Can you work these out from the model? Positions are in its coordinate system, mm. A direction names the side the tool comes from. Round coordinates to 2 decimals unless told otherwise and drop trailing zeros. Order: outer loops, then holes, each group sorted by start corner. A loop starts at its lowest first (then second) coordinate and runs counter-clockwise, first axis right, second up. Notation, with made-up numbers: (-5.5, 75) -> (32.5, 75) arc R22 cw to (32.5, 88) -> close; hole circle Ø2 at (-26, -11.5). An arc over 180 degrees is marked (long way). One line per item, written item: value.
```python
from build123d import *

# Parameters (mm, degrees)
SKETCH1_R           = 2
EXTRUDE1_DEPTH      = 8
CUT_SWEEP1_PITCH    = 0.7
SKETCH6_R           = 3.5
EXTRUDE2_DEPTH      = 4
CUT_EXTRUDE1_DEPTH  = 2.25
CHAMFER1_SIZE       = 0.35
SKETCH10_R          = 2
BOSS_EXTRUDE1_DEPTH = 8
CHAMFER2_SIZE       = 0.5
CHAMFER2_SIZE2      = 0.866025404


with BuildPart() as part:
    # Sketch1 → Extrude1 (new body)
    with BuildSketch(Plane.XY):
        Circle(SKETCH1_R)
    extrude(amount=-EXTRUDE1_DEPTH)

    # Cut-Sweep1: the profile of Sketch3 profile screwed along a right-hand helix of 12.428571 turns, 6 arcs to a turn; built about Z, then put on its axis
    cut_sweep1_z = Axis((0, 0, 0), (0, 0, 1))
    cut_sweep1_corners = [(2.0003, 0, -0.612673205), (1.545336663, 0, -0.35), (1.545336663, 0, -0.2625), (2.0003, 0, 0.000173205)]
    with BuildLine(mode=Mode.PRIVATE) as cut_sweep1_profile:
        Line(cut_sweep1_corners[0], cut_sweep1_corners[1])
        Line(cut_sweep1_corners[1], cut_sweep1_corners[2])
        Line(cut_sweep1_corners[2], cut_sweep1_corners[3])
        Line(cut_sweep1_corners[3], cut_sweep1_corners[0])
    cut_sweep1_cap = Face(cut_sweep1_profile.wire())
    cut_sweep1_turn_angles = [0, 30, 60, 90, 120, 150, 180, 210, 240, 270, 300, 330, 360]
    cut_sweep1_turn_weights = [1, 0.8660254037844387, 1, 0.8660254037844387, 1, 0.8660254037844387, 1, 0.8660254037844387, 1, 0.8660254037844387, 1, 0.8660254037844387, 1]
    cut_sweep1_turn_rails = [Edge.make_bspline([Vector(p[0], p[1], 0).rotate(cut_sweep1_z, cut_sweep1_turn_angles[k]) / cut_sweep1_turn_weights[k] + Vector(0, 0, p[2] + CUT_SWEEP1_PITCH * cut_sweep1_turn_angles[k] / 360) for k in range(13)], [0, 0, 0, 1, 1, 2, 2, 3, 3, 4, 4, 5, 5, 6, 6, 6], 2, cut_sweep1_turn_weights) for p in cut_sweep1_corners]
    cut_sweep1_turn_sides = [Face.make_surface_from_curves(cut_sweep1_turn_rails[p[0]], cut_sweep1_turn_rails[p[1]]) for p in [(0, 1), (1, 2), (2, 3), (3, 0)]]
    cut_sweep1_last_angles = [4320, 4350, 4380, 4410, 4440, 4457.142857143, 4474.285714286]
    cut_sweep1_last_weights = [1, 0.8660254037844387, 1, 0.8660254037844387, 1, 0.9555728057861561, 1]
    cut_sweep1_last_rails = [Edge.make_bspline([Vector(p[0], p[1], 0).rotate(cut_sweep1_z, cut_sweep1_last_angles[k]) / cut_sweep1_last_weights[k] + Vector(0, 0, p[2] + CUT_SWEEP1_PITCH * cut_sweep1_last_angles[k] / 360) for k in range(7)], [0, 0, 0, 1, 1, 2, 2, 3, 3, 3], 2, cut_sweep1_last_weights) for p in cut_sweep1_corners]
    cut_sweep1_last_sides = [Face.make_surface_from_curves(cut_sweep1_last_rails[p[0]], cut_sweep1_last_rails[p[1]]) for p in [(0, 1), (1, 2), (2, 3), (3, 0)]]
    cut_sweep1 = Plane(origin=(0, 0, 0), x_dir=(0, 1, 0), z_dir=(0, 0, -1)) * Solid(Shell([*[p.moved(Location((0, 0, CUT_SWEEP1_PITCH * i))) for i in range(12) for p in cut_sweep1_turn_sides], *cut_sweep1_last_sides, cut_sweep1_cap, cut_sweep1_cap.rotate(cut_sweep1_z, 4474.285714286).moved(Location((0, 0, CUT_SWEEP1_PITCH * 4474.285714286 / 360)))]))
    add(cut_sweep1, mode=Mode.SUBTRACT)

    # Sketch4 → Cut-Revolve1 (revolve, cut)
    with BuildSketch(Plane(origin=(0, 0, 0), x_dir=(0, 0, -1), z_dir=(1, 0, 0)), mode=Mode.PRIVATE) as cut_revolve1_sk:
        Polygon((0.496211411, 2), (0, 1.291336663), (0, 2), align=None)
    revolve(cut_revolve1_sk.sketch.rotate(Axis((0, 0, 0), (0, 0, -1)), 271.401126896), axis=Axis((0, 0, 0), (0, 0, -1)), mode=Mode.SUBTRACT)

    # Sketch6 → Extrude2 (add)
    with BuildSketch(Plane(origin=(0, 0, -8), x_dir=(-1, 0, 0), z_dir=(0, 0, -1))):
        Circle(SKETCH6_R)
    extrude(amount=EXTRUDE2_DEPTH)

    # Sketch7 → Cut-Extrude1 (cut)
    with BuildSketch(Plane(origin=(0, 0, -12), x_dir=(-1, 0, 0), z_dir=(0, 0, -1))):
        Polygon((0, 1.732050808), (-1.5, 0.866025404), (-1.5, -0.866025404), (0, -1.732050808), (1.5, -0.866025404), (1.5, 0.866025404), align=None)
    extrude(amount=-CUT_EXTRUDE1_DEPTH, mode=Mode.SUBTRACT)

    # Cut-Extrude2 cone 1 section (through the dimple's axis) → Cut-Extrude2 (revolve, cut)
    with BuildSketch(Plane(origin=(0, 0, -12), x_dir=(0, 1, 0), z_dir=(1, 0, 0))):
        Polygon((0, 0), (1.732050808, 0), (0, 1.732050808), align=None)
    revolve(axis=Axis((0, 0, -12), (0, 0, 1)), mode=Mode.SUBTRACT)

    # Chamfer1
    chamfer1_edges = [part.edges().sort_by_distance(p)[0] for p in [
        (3.5, 0, -8),
        (3.5, 0, -12),
    ]]
    chamfer(chamfer1_edges, length=CHAMFER1_SIZE)

    # Sketch10 → Boss-Extrude1 (add)
    with BuildSketch(Plane.XY):
        Circle(SKETCH10_R)
    extrude(amount=-BOSS_EXTRUDE1_DEPTH)

    # Chamfer2
    chamfer2_edges = [part.edges().sort_by_distance(p)[0] for p in [
        (-2, 0, 0),
    ]]
    chamfer2_side = [part.faces().sort_by_distance(p)[0] for p in [
        (-2, 0, -4),
    ]]
    chamfer(chamfer2_edges, length=CHAMFER2_SIZE, length2=CHAMFER2_SIZE2, reference=chamfer2_side[0])


solid = part.part
```
Q1. We'd pull the mould along Y, two halves only. Please class faces 3 (the face through (0, 0, -9.75)), 4 (the face through (0, -2, -4)), 5 (the face through (-1, -2, -8)): released by +Y, released by -Y, zero draft, split by the parting line, or undercut.
Answers below:
face 3: undercut
face 4: split by the parting line
face 5: zero draft
Q2. I want a section at A-A on y = 0. List the corners of the cut face in (x, z) for me.
Answers below:
outline: (-3.5, -11.65) -> (-3.15, -12) -> (-1.73, -12) -> (-1.5, -11.77) -> (-1.5, -9.75) -> (1.5, -9.75) -> (1.5, -11.77) -> (1.73, -12) -> (3.15, -12) -> (3.5, -11.65) -> (3.5, -8.35) -> (3.15, -8) -> (2, -8) -> (2, -0.5) -> (1.13, 0) -> (-1.13, 0) -> (-2, -0.5) -> (-2, -8) -> (-3.15, -8) -> (-3.5, -8.35) -> close
Q3. Please list where these lines run through material, in increasing order: line 1 along Z through (x, y) = (-0.75, 3); line 2 along X through (y, z) = (-1, -7); line 3 along X through (y, z) = (3, -11).
Answers below:
line 1: -12 to -8
line 2: -1.73 to 1.73
line 3: -1.8 to 1.8
Q4. Will these pins go through, and if not, where does the flat tip stop? pin 1 Ø2 at (y, z) = (0.5, -6.5) entering from -X; pin 2 Ø4 at (y, z) = (-2.5, -9) entering from +X; pin 3 Ø4 at (y, z) = (2.5, -1.5) entering from +X.
Answers below:
pin 1: x = -2
pin 2: x = 3.46
pin 3: x = 1.94
Q5. On a 3-axis mill with a long thin cutter (end or side, diameter ignored), from which of +Z, -Z, +X, -X, +Y, -Y can I reach the whole of each face in a straight line? I mean faces 1 (the face through (1.5, 0, -11)), 2 (the face through (0, 0, 0)). Say none if no direction works.
Answers below:
face 1: -Z
face 2: +Z, +X, -X, +Y, -Y
Q6. I want a section at B-B on z = -10. List the corners of the cut face in (x, y) for me, plus the area to 3 significant figures.
Answers below:
outline: circle Ø7 at (0, 0); hole (-1.5, -0.87) -> (0, -1.73) -> (1.5, -0.87) -> (1.5, 0.87) -> (0, 1.73) -> (-1.5, 0.87) -> close
area: 30.7 mm^2
Q7. I want a section at C-C on z = -3.5. List the corners of the cut face in (x, y) for me, plus the area to 3 significant figures.
Answers below:
outline: circle Ø4 at (0, 0)
area: 12.6 mm^2
